from build123d import *

# Parameters (mm, degrees)
F0_R     = 1
F0_R_2   = 2
F1_DEPTH = 1.5


with BuildPart() as f1:
    # F0 (on Top) → F1 (new body)
    with BuildSketch(Plane.XY):
        with BuildLine():
            ThreePointArc((4, 0), (0, -4), (-4, 0))
            Line((-4, 0), (-4, 2.5))
            Line((-4, 2.5), (-8.5, 2.5))
            Line((-8.5, 2.5), (-8.5, -13.5))
            Line((-8.5, -13.5), (18.5, -13.5))
            Line((18.5, -13.5), (18.5, 2.5))
            Line((18.5, 2.5), (4, 2.5))
            Line((4, 2.5), (4, 0))
        make_face()
        with Locations((0, -6)):
            Circle(F0_R, mode=Mode.SUBTRACT)
        with Locations((15, -10)):
            Circle(F0_R_2, mode=Mode.SUBTRACT)
        with Locations((-4.242641, -4.242641)):
            Circle(F0_R, mode=Mode.SUBTRACT)
        with Locations((4.242641, -4.242641)):
            Circle(F0_R, mode=Mode.SUBTRACT)
        with Locations((-6, 0)):
            Circle(F0_R, mode=Mode.SUBTRACT)
        with Locations((6, 0)):
            Circle(F0_R, mode=Mode.SUBTRACT)
    extrude(amount=F1_DEPTH)


solid = f1.part
Here's how the part is built. I have some questions about the finished solid (model axes, mm). A direction names the side the tool comes from. Round coordinates to 2 decimals unless told otherwise and drop trailing zeros. Loops run counter-clockwise (first coordinate to the right, second up) from the corner with the lowest first, then second, coordinate; pieces in that order, holes last. Notation, with made-up numbers: M 64,47.5 L 91,47.5 A17 cw 91,64.5 Z; hole C 82,67 d7. An arc over 180 degrees is marked long. Write each question's results on one line, items separated by ' | '. Start each with the question number.
(1) I want a section at C-C (y = -3.5). Please give me the cut outline in (x, z).
(2) If I drill on probe 1 along X at (y, z) = (-3.5, 0.85); probe 2 along Y at (x, z) = (6, 1.05); probe 3 along X at (y, z) = (0.5, 1.4), over which ranges is the centre line in solid material (lowest first)? Write a range as from..to.
(3) I want a section at B-B (y = -6). Please give me the cut outline in (x, z), then the cut area to 3 significant figures.
(4) I want a section at A-A (x = 0). Please give me the cut outline in (y, z), then the cut area to 4 significant figures.
(5) Thinking about a two-plate mould opening in Y: for faces 3 (the cylindrical face through (13.526, -8.648, 0.74)), 4 (the cylindrical face through (0, -4, 1)), 5 (the flat face through (5, -13.5, 1)), which applies, pulls with the +Y half, pulls with the -Y half, needs draft (parallel to the pull), parting line crosses it, or undercut?
(6) On a 3-axis mill with a long thin cutter (end or side, diameter ignored), from which of +Z, -Z, +X, -X, +Y, -Y can I reach the whole of each face in a straight line? I mean faces 1 (the flat face through (4, 1, 1)), 2 (the cylindrical face through (-6.8, -0.6, 0.7)). Say none if no direction works.
(7) I want a section at D-D (z = 1.05). Please give me the cut outline in (x, y).
Solved:
1) outline: M -8.5,0 L -4.91,0 L -4.91,1.5 L -8.5,1.5 Z; M -3.57,0 L -1.94,0 L -1.94,1.5 L -3.57,1.5 Z; M 1.94,0 L 3.57,0 L 3.57,1.5 L 1.94,1.5 Z; M 4.91,0 L 18.5,0 L 18.5,1.5 L 4.91,1.5 Z
2) probe 1: x = -8.5..-4.91, -3.57..-1.94, 1.94..3.57, 4.91..18.5 | probe 2: y = -13.5..-1, 1..2.5 | probe 3: x = -8.5..-6.87, -5.13..-4, 4..5.13, 6.87..18.5
3) outline: M -8.5,0 L -1,0 L -1,1.5 L -8.5,1.5 Z; M 1,0 L 18.5,0 L 18.5,1.5 L 1,1.5 Z | area: 37.5 mm²
4) outline: M -13.5,0 L -7,0 L -7,1.5 L -13.5,1.5 Z; M -5,0 L -4,0 L -4,1.5 L -5,1.5 Z | area: 11.25 mm²
5) face 3: undercut | face 4: pulls with the +Y half | face 5: pulls with the -Y half
6) face 1: +Z, -Z, +Y | face 2: +Z, -Z
7) outline: M -8.5,-13.5 L 18.5,-13.5 L 18.5,2.5 L 4,2.5 L 4,0 A4 cw -4,0 L -4,2.5 L -8.5,2.5 Z; hole C -6,0 d2; hole C -4.24,-4.24 d2; hole C 0,-6 d2; hole C 4.24,-4.24 d2; hole C 6,0 d2; hole C 15,-10 d4
